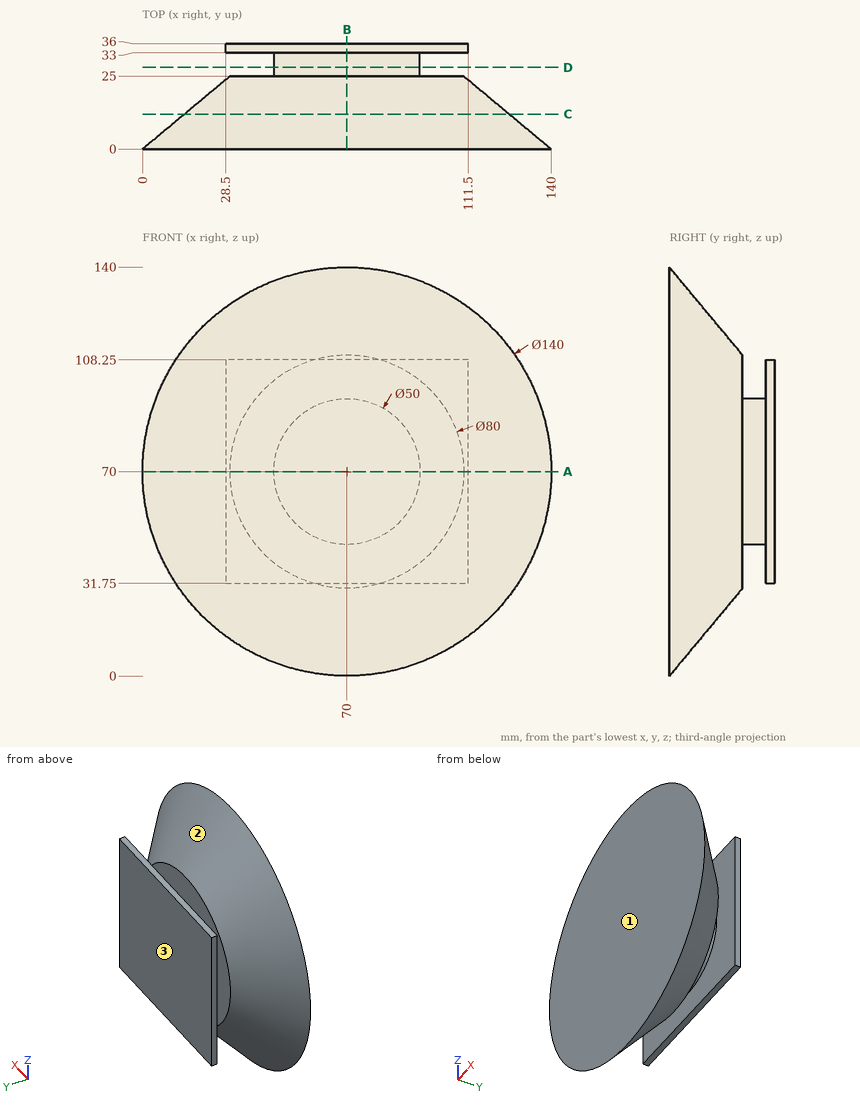
Geometry check sheet. Reference: drawing and pictorial views, mm from the part's lowest x, y, z. Give positions to 0.01 mm unless a question says otherwise; leave off trailing zeros. Loops run counter-clockwise (first coordinate to the right, second up) from the corner with the lowest first, then second, coordinate; pieces in that order, holes last. Notation, with made-up numbers: (79.25, 43.25) - (112.25, 43.25) arc R21 cw to (112.25, 61.25) - close; hole circle Ø9 at (17, 23.25). An arc over 180 degrees is marked (long way). One line per question, with ' | ' between items. Start each with the question number.
1. Cross-section at B-B, the plane x = 70. Enter the section's corners in (y, z).
2. Material ranges on line 1 along Y through (x, z) = (100.5, 86); line 2 along X through (y, z) = (34.5, 65); line 3 along Y through (x, z) = (103.5, 103.5), recorded low to high. Write a range as [from, to].
3. Draft check along Y on the marked faces 1, 2 and 3. Enter one of: released by +Y, released by -Y, zero draft, split by the parting line, or undercut.
4. Cross-section at C-C, the plane y = 12. Enter the section's corners in (x, z).
5. Cross-section at A-A, the plane z = 70. Enter the section's corners in (x, y), plus the area to 3 significant figures.
6. Cross-section at D-D, the plane y = 28. Enter the section's corners in (x, z).
7. Gauge pin test, flat ends, axial feed: pin 1 Ø10 at (y, z) = (9.5, 62.5) entering from -X; pin 2 Ø3.5 at (x, y) = (84, 34) entering from +Z; pin 3 Ø8 at (x, y) = (72.5, 23.5) entering from -Z. Record the tip position at first contact, or that the pin passes through.
Check result:
1) outline: (0, 0) - (25, 30) - (25, 45) - (33, 45) - (33, 31.75) - (36, 31.75) - (36, 108.25) - (33, 108.25) - (33, 95) - (25, 95) - (25, 110) - (0, 140) - close
2) line 1: y = [0, 25], [33, 36] | line 2: x = [28.5, 111.5] | line 3: y = [0, 18.85], [33, 36]
3) face 1: released by -Y | face 2: undercut | face 3: released by +Y
4) outline: circle Ø111.2 at (70, 70)
5) outline: (0, 0) - (140, 0) - (110, 25) - (95, 25) - (95, 33) - (111.5, 33) - (111.5, 36) - (28.5, 36) - (28.5, 33) - (45, 33) - (45, 25) - (30, 25) - close | area: 3,400 mm2
6) outline: circle Ø50 at (70, 70)
7) pin 1: stops at x = 5.81 | pin 2: stops at z = 108.25 | pin 3: stops at z = 23.46
